Source: CAD feature listing. Evaluate the final solid. Frame: model axes, mm. Face numbers are marked on the shaded views. A direction names the side the tool comes from. Coordinates: 2 decimals unless noted, no trailing zeros. Order: outer loops, then holes, each group sorted by start corner. A loop starts at its lowest first (then second) coordinate and runs counter-clockwise, first axis right, second up.
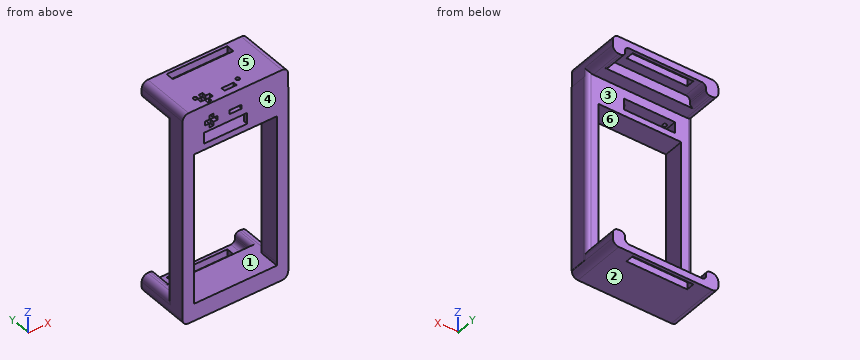
```python
from build123d import *

# Parameters (mm, degrees)
SKETCH_1_W               = 52.13
SKETCH_1_H               = 16.25
SKETCH_1_R               = 0.95
EXTRUDE_1_DEPTH          = 10
SKETCH_2_W               = 7.1
SKETCH_2_H               = 10
EXTRUDE_2_DEPTH          = 11.95
EXTRUDE_3_DEPTH          = 10.6
SKETCH_4_W               = 30
SKETCH_4_H               = 4
CUT_EXTRUDE_1_DEPTH      = 11
SKETCH_6_W               = 5.65
SKETCH_6_H               = 10
EXTRUDE_4_DEPTH          = 80
CUT_EXTRUDE_2_DEPTH      = 80
CUT_EXTRUDE_2_DEPTH_BACK = 6.25
SKETCH_7_W               = 52.13
SKETCH_7_H               = 1.45
SKETCH_7_H_2             = 1.85
SKETCH_8_W               = 11.056524021
SKETCH_8_H               = 11.95
CUT_EXTRUDE_3_DEPTH      = 103.005836269
SKETCH_9_W               = 3.1
SKETCH_9_H               = 10
EXTRUDE_5_DEPTH          = 25.2
SKETCH_10_W              = 2
SKETCH_10_H              = 2
EXTRUDE_6_DEPTH          = 8.85
SKETCH_11_W              = 40.93148405
SKETCH_11_H              = 1.45
CUT_EXTRUDE_4_DEPTH      = 103.005836269
SKETCH_12_W              = 5.73041858
SKETCH_12_H              = 11.95
EXTRUDE_7_DEPTH          = 10
FILLET_1_R               = 3
FILLET_2_R               = 2
SKETCH_13_R              = 1.05
CUT_EXTRUDE_5_DEPTH      = 105.087334213
FILLET_3_R               = 2
SKETCH_14_R              = 0.95
EXTRUDE_8_DEPTH          = 3.4
SKETCH_15_W              = 23.6
SKETCH_15_H              = 5.45
SKETCH_15_W_2            = 1.6
EXTRUDE_9_DEPTH          = 10
SKETCH_15_3_W            = 23.6
SKETCH_15_3_H            = 5.45
SKETCH_15_3_W_2          = 1.6
CUT_EXTRUDE_6_DEPTH      = 103.005836318
SKETCH_16_W              = 2
SKETCH_16_H              = 5.45
EXTRUDE_10_DEPTH         = 2
EXTRUDE_START            = -13.4
SKETCH_17_R              = 0.95
EXTRUDE_11_DEPTH         = 13.4
SKETCH_17_4_R            = 0.95
SKETCH_17_4_R_2          = 1.05
EXTRUDE_12_DEPTH         = 8.55
CUT_EXTRUDE_7_REACH      = 114.071
SKETCH_18_R              = 0.95
SKETCH_19_R              = 0.95
EXTRUDE_13_DEPTH         = 8.55
SKETCH_20_W              = 6
SKETCH_20_H              = 2
SKETCH_20_W_2            = 2
SKETCH_20_H_2            = 6
CUT_EXTRUDE_1_2_DEPTH    = 2
SKETCH_21_W              = 6
SKETCH_21_H              = 2
SKETCH_21_W_2            = 2
SKETCH_21_H_2            = 6
CUT_EXTRUDE_2_2_DEPTH    = 2


with BuildPart() as part:
    # 草图1 → 凸台-拉伸1 (new body)
    with BuildSketch(Plane.XY):
        with Locations((6.365, 2.125)):
            Rectangle(SKETCH_1_W, SKETCH_1_H)
        with Locations((-10.5, 0)):
            Circle(SKETCH_1_R, mode=Mode.SUBTRACT)
        with Locations(Location((10.5, 0, 0), (0, 0, 180))):
            Circle(SKETCH_1_R, mode=Mode.SUBTRACT)
    extrude_1 = extrude(amount=EXTRUDE_1_DEPTH)

    # 草图2 → 凸台-拉伸2 (add)
    with BuildSketch(Plane(origin=(0, 0, 0), x_dir=(-1, 0, 0), z_dir=(0, 0, -1))):
        with Locations((16.15, -1)):
            Rectangle(SKETCH_2_W, SKETCH_2_H)
        with Locations((-16.15, -1)):
            Rectangle(SKETCH_2_W, SKETCH_2_H)
    extrude_2 = extrude(amount=EXTRUDE_2_DEPTH)

    # 草图3 → 凸台-拉伸3 (add)
    with BuildSketch(Plane(origin=(0, 10.25, 0), x_dir=(1, 0, 0), z_dir=(0, 1, 0))):
        Polygon((32.43, -10), (-19.7, -10), (-19.7, -1.45), (-13.635, -1.45), (-13.635, -6.45), (26.365, -6.45), (26.365, -1.45), (32.43, -1.45), align=None)
    extrude_3 = extrude(amount=EXTRUDE_3_DEPTH)

    # 草图4 → Cut-Extrude 1 (cut)
    with BuildSketch(Plane.XY.offset(10)):
        with Locations((6.41520929, 17.24732554)):
            Rectangle(SKETCH_4_W, SKETCH_4_H)
    cut_extrude_1 = extrude(amount=-CUT_EXTRUDE_1_DEPTH, mode=Mode.SUBTRACT)

    # 草图6 → 凸台-拉伸4 (add)
    with BuildSketch(Plane(origin=(0, 0, -11.95), x_dir=(-1, 0, 0), z_dir=(0, 0, -1))):
        with Locations((16.875, -1)):
            Rectangle(SKETCH_6_W, SKETCH_6_H)
    extrude_4 = extrude(amount=EXTRUDE_4_DEPTH)

    # 镜向1: 凸台-拉伸2, 凸台-拉伸4 across plane
    add(extrude_2.mirror(Plane.ZY.offset(-6.41520929)))
    add(extrude_4.mirror(Plane.ZY.offset(-6.41520929)))

    # 镜向2: 凸台-拉伸1, 凸台-拉伸3, Cut-Extrude 1 across plane
    add(extrude_1.mirror(Plane.XY.offset(-42.6)))
    add(extrude_3.mirror(Plane.XY.offset(-42.6)))
    add(cut_extrude_1.mirror(Plane.XY.offset(-42.6)), mode=Mode.SUBTRACT)

    # 草图7 → Cut-Extrude 2 (cut, two sides: drawn at the far end of the back side and taken through both)
    with BuildSketch(Plane(origin=(0, 10.25, 0), x_dir=(1, 0, 0), z_dir=(0, 1, 0)).offset(-CUT_EXTRUDE_2_DEPTH_BACK)):
        with Locations((6.365, -0.725)):
            Rectangle(SKETCH_7_W, SKETCH_7_H)
        with Locations((6.365, 85.725)):
            Rectangle(SKETCH_7_W, SKETCH_7_H_2)
    extrude(amount=CUT_EXTRUDE_2_DEPTH + CUT_EXTRUDE_2_DEPTH_BACK, mode=Mode.SUBTRACT)

    # 草图8 → 切除-拉伸3 (cut, through all)
    with BuildSketch(Plane(origin=(0, 4, 0), x_dir=(1, 0, 0), z_dir=(0, 1, 0))):
        with Locations((-1.34131941, 5.975)):
            Rectangle(SKETCH_8_W, SKETCH_8_H)
    extrude(amount=-CUT_EXTRUDE_3_DEPTH, mode=Mode.SUBTRACT)

    # 草图9 → 凸台-拉伸5 (add)
    with BuildSketch(Plane.ZY.offset(-12.6)):
        with Locations((-10.4, -1)):
            Rectangle(SKETCH_9_W, SKETCH_9_H)
    extrude(amount=EXTRUDE_5_DEPTH)

    # 草图10 → 凸台-拉伸6 (add)
    with BuildSketch(Plane(origin=(0, 0, 0), x_dir=(-1, 0, 0), z_dir=(0, 0, -1))):
        with Locations((-11.6, -5)):
            Rectangle(SKETCH_10_W, SKETCH_10_H)
        with Locations((11.6, -5)):
            Rectangle(SKETCH_10_W, SKETCH_10_H)
    extrude(amount=EXTRUDE_6_DEPTH)

    # 草图11 → 切除-拉伸4 (cut, through all)
    with BuildSketch(Plane(origin=(0, 4, 0), x_dir=(1, 0, 0), z_dir=(0, 1, 0))):
        with Locations((6.415742025, 85.925)):
            Rectangle(SKETCH_11_W, SKETCH_11_H)
    extrude(amount=-CUT_EXTRUDE_4_DEPTH, mode=Mode.SUBTRACT)

    # 草图12 → 凸台-拉伸7 (add)
    with BuildSketch(Plane(origin=(0, 4, 0), x_dir=(1, 0, 0), z_dir=(0, 1, 0))):
        with Locations((22.56520929, 5.975)):
            Rectangle(SKETCH_12_W, SKETCH_12_H)
    extrude(amount=-EXTRUDE_7_DEPTH)

    # 圆角1
    fillet_1_edges = [part.edges().sort_by_distance(p)[0] for p in [
        (32.43, 7.425, 10),
        (-19.7, 7.425, -95.2),
        (32.43, 7.425, -95.2),
        (-19.7, 12.425, -86.65),
        (32.43, 12.425, -86.65),
        (-19.7, 7.425, 10),
        (-19.7, 12.425, 1.45),
        (32.43, 12.425, 1.45),
    ]]
    fillet(fillet_1_edges, radius=FILLET_1_R)

    # 圆角2
    fillet_2_edges = [part.edges().sort_by_distance(p)[0] for p in [
        (32.53041858, 4, -45.975),
        (-19.7, 4, -42.6),
    ]]
    fillet(fillet_2_edges, radius=FILLET_2_R)

    # 草图13 → 切除-拉伸5 (cut, through all)
    with BuildSketch(Plane(origin=(0, 0, 1.45), x_dir=(-1, 0, 0), z_dir=(0, 0, -1))):
        with Locations((0, 5.05)):
            Circle(SKETCH_13_R)
    extrude(amount=-CUT_EXTRUDE_5_DEPTH, mode=Mode.SUBTRACT)

    # 圆角3
    fillet_3_edges = [part.edges().sort_by_distance(p)[0] for p in [
        (-13.635, 15.55, -86.65),
        (-13.635, 15.55, -91.65),
        (26.365, 15.55, -91.65),
        (26.365, 15.55, -86.65),
        (26.365, 15.55, 1.45),
        (26.365, 15.55, 6.45),
        (-13.635, 15.55, 6.45),
        (-13.635, 15.55, 1.45),
    ]]
    fillet(fillet_3_edges, radius=FILLET_3_R)

    # 草图14 → 凸台-拉伸8 (add)
    with BuildSketch(Plane(origin=(0, 0, 0), x_dir=(-1, 0, 0), z_dir=(0, 0, -1))):
        Polygon((10.6, -4), (12.6, -4), (12.6, 4), (-12.6, 4), (-12.6, -4), (-10.6, -4), (-10.6, -6), (10.6, -6), align=None)
        with Locations((-10.5, 0)):
            Circle(SKETCH_14_R, mode=Mode.SUBTRACT)
        with Locations((10.5, 0)):
            Circle(SKETCH_14_R, mode=Mode.SUBTRACT)
    extrude(amount=EXTRUDE_8_DEPTH)

    # 草图15 → 凸台-拉伸9 (add, through all)
    with BuildSketch(Plane(origin=(0, 4, 0), x_dir=(1, 0, 0), z_dir=(0, 1, 0))):
        with Locations((0.8, 6.125)):
            Rectangle(SKETCH_15_W, SKETCH_15_H)
        with Locations((-11.8, 6.125)):
            Rectangle(SKETCH_15_W_2, SKETCH_15_H)
        with Locations((13.4, 6.125)):
            Rectangle(SKETCH_15_W_2, SKETCH_15_H)
    extrude(amount=-EXTRUDE_9_DEPTH)

    # 草图15<3> → 切除-拉伸6 (cut, through all)
    with BuildSketch(Plane(origin=(0, 4, 0), x_dir=(1, 0, 0), z_dir=(0, 1, 0))):
        with Locations((0.8, 6.125)):
            Rectangle(SKETCH_15_3_W, SKETCH_15_3_H)
        with Locations((13.4, 6.125)):
            Rectangle(SKETCH_15_3_W_2, SKETCH_15_3_H)
    extrude(amount=-CUT_EXTRUDE_6_DEPTH, mode=Mode.SUBTRACT)

    # 草图16 → 凸台-拉伸10 (add)
    with BuildSketch(Plane(origin=(0, -6, 0), x_dir=(-1, 0, 0), z_dir=(0, -1, 0))):
        with Locations((10, 6.125)):
            Rectangle(SKETCH_16_W, SKETCH_16_H)
        with Locations((-13.2, 6.125)):
            Rectangle(SKETCH_16_W, SKETCH_16_H)
    extrude(amount=-EXTRUDE_10_DEPTH)

    # 草图17 → 凸台-拉伸11 (add)
    with BuildSketch(Plane.XY.offset(10).offset(EXTRUDE_START)):
        with Locations((-10.5, 0)):
            Circle(SKETCH_17_R)
        with Locations(Location((10.5, 0, 0), (0, 0, 180))):
            Circle(SKETCH_17_R)
    extrude(amount=EXTRUDE_11_DEPTH)

    # 草图17<4> → 凸台-拉伸12 (add)
    with BuildSketch(Plane.XY.offset(10)):
        with Locations(Location((10.5, 0, 0), (0, 0, 180))):
            Circle(SKETCH_17_4_R)
        with Locations((0, 5.05)):
            Circle(SKETCH_17_4_R_2)
        with Locations((-10.5, 0)):
            Circle(SKETCH_17_4_R)
    extrude(amount=-EXTRUDE_12_DEPTH)

    # 草图18 → 切除-拉伸7 (cut, up to next)
    with BuildSketch(Plane.XY.offset(10), mode=Mode.PRIVATE) as cut_extrude_7_sk1:
        with Locations((12.1, 0)):
            Circle(SKETCH_18_R)
    cut_extrude_7_tool1 = extrude(cut_extrude_7_sk1.sketch, amount=-CUT_EXTRUDE_7_REACH, mode=Mode.PRIVATE) & part.part
    # 草图18 → 切除-拉伸7 (cut, up to next)
    with BuildSketch(Plane.XY.offset(10), mode=Mode.PRIVATE) as cut_extrude_7_sk2:
        with Locations((-8.9, 0)):
            Circle(SKETCH_18_R)
    cut_extrude_7_tool2 = extrude(cut_extrude_7_sk2.sketch, amount=-CUT_EXTRUDE_7_REACH, mode=Mode.PRIVATE) & part.part
    add(cut_extrude_7_tool1.solids().sort_by_distance((12.1, 0, 10))[0], mode=Mode.SUBTRACT)
    add(cut_extrude_7_tool2.solids().sort_by_distance((-8.9, 0, 10))[0], mode=Mode.SUBTRACT)

    # 草图19 → 凸台-拉伸13 (add, through all)
    with BuildSketch(Plane.XY.offset(-86.65)):
        with Locations((-10.5, 0)):
            Circle(SKETCH_19_R)
        with Locations((10.5, 0)):
            Circle(SKETCH_19_R)
    extrude(amount=-EXTRUDE_13_DEPTH)

    # 草图20 → Cut-Extrude 1 2 (cut)
    with BuildSketch(Plane.XZ.offset(6)):
        with Locations((-5.5, 1)):
            Rectangle(SKETCH_20_W, SKETCH_20_H)
        with Locations((-5.5, 1)):
            Rectangle(SKETCH_20_W_2, SKETCH_20_H_2)
        with Locations((6.5, 1)):
            Rectangle(SKETCH_20_W, SKETCH_20_H)
    extrude(amount=-CUT_EXTRUDE_1_2_DEPTH, mode=Mode.SUBTRACT)

    # 草图21 → Cut-Extrude 2 2 (cut)
    with BuildSketch(Plane.XY.offset(10)):
        with Locations((-5.5, -2)):
            Rectangle(SKETCH_21_W, SKETCH_21_H)
        with Locations((-5.5, -2)):
            Rectangle(SKETCH_21_W_2, SKETCH_21_H_2)
        with Locations((6.3, -2)):
            Rectangle(SKETCH_21_W, SKETCH_21_H)
    extrude(amount=-CUT_EXTRUDE_2_2_DEPTH, mode=Mode.SUBTRACT)


solid = part.part
```
1. Section query C-C, the plane x = -3.5. Count the separate pieces of the cut face and the enclosed holes in it, plus the area to 3 significant figures.
2. Draft query along Z for the marked faces 1, 2, 3 and 4. Return one class per face: +Z half, -Z half, draft (parallel to the pull), parting line (faces both ways), or undercut.
3. Material intervals for line 1 along Z through (x, y) = (-6.5, -2); line 2 along Z through (x, y) = (8.5, 3.5); line 3 along Y through (x, z) = (12.1, 3), sorted ascending.
4. Contact query for flat-ended pins moving along their axis: P1, Ø2, axis at x = 13, z = -6, coming from the +Y side; P2, Ø1.1, axis at y = 17.5, z = 7.5, coming from the +X side; P3, Ø1, axis at x = 22, z = -4, coming from the +Y side. Output: stop coordinate, or through.
5. Access query for the marked faces 5 and 6. Directions: +Z, -Z, +X, -X, +Y, -Y. A direction counts if a zero-diameter tool reaches every point of the face in a straight line with its end or side. Return the directions, or none.
6. Section query D-D, the plane x = 16. Output: boundary loops of the cut face in (y, z), plus the area to 3 significant figures.
7. Section query B-B, the plane z = -39.5. Output: boundary loops of the cut face in (x, y), plus the area to 3 significant figures.
Answer key:
1. separate pieces: 5
1. enclosed holes: 0
1. area: 396 mm2
2. face 1: undercut
2. face 2: -Z half
2. face 3: undercut
2. face 4: draft
3. line 1: z = -95.2 to -86.65, -11.95 to -8.85, -3.4 to 8
3. line 2: z = -95.2 to -86.65, -11.95 to -8.85, -3.4 to 10
3. line 3: y = -6 to -0.95, 0.95 to 10.25
4. P1: stops at y = -4
4. P2: stops at x = 32.43
4. P3: stops at y = 4
5. face 5: +Z, +X, -X, +Y, -Y
5. face 6: +Y, -Y
6. outline: (-6, -95.2) - (15.25, -95.2) - (15.25, -91.65) - (10.25, -91.65) - (10.25, -86.65) - (-6, -86.65) - close; (-6, -11.95) - (4, -11.95) - (4, 1.45) - (10.25, 1.45) - (10.25, 6.45) - (15.25, 6.45) - (15.25, 10) - (-6, 10) - close; (19.25, -95.2) - (20.85, -95.2) - (20.85, -91.65) - (19.25, -91.65) - close; (19.25, 6.45) - (20.85, 6.45) - (20.85, 10) - (19.25, 10) - close
6. area: 459 mm2
7. outline: (-19.7, -6) - (-14.05, -6) - (-14.05, 4) - (-17.7, 4) arc R2 ccw to (-19.7, 2) - close; (26.88, -6) - (32.53, -6) - (32.53, 2) arc R2 ccw to (30.53, 4) - (26.88, 4) - close
7. area: 111 mm2
